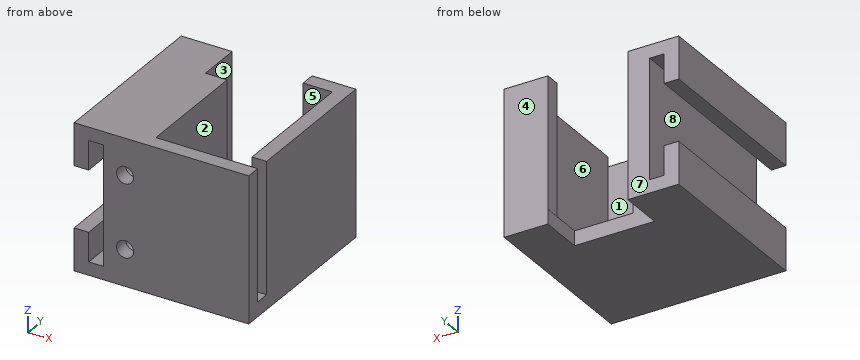
Autodesk Inventor part; units mm, degrees
ref_plane "YZ Plane" through (0, 0, 0) normal (1, 0, 0) x (0, 1, 0)
ref_plane "XZ Plane" through (0, 0, 0) normal (0, 1, 0) x (-1, 0, 0)
ref_plane "XY Plane" through (0, 0, 0) normal (0, 0, 1) x (1, 0, 0)
sketch "Sketch3" plane through (0, 0, 0) normal (0, 0, 1) x (1, 0, 0)
  line L0 (0, 0) -> (0, 60)
  line L1 (0, 60) -> (17.5, 60)
  line L2 (17.5, 60) -> (17.5, 45)
  line L3 (17.5, 45) -> (45, 45)
  line L4 (45, 45) -> (45, 60)
  line L5 (10.4377, 0) -> (0, 0)
  line L6 (45, 60) -> (60, 60)
  line L7 (60, 60) -> (60, 0)
  line L8 (60, 0) -> (0, 0)
  dimension "d7" = 60
  dimension "d8" = 17.5
  dimension "d12" = 15
  dimension "d13" = 27.5
  dimension "d14" = 15
  dimension "d15" = 60
  dimension "d16" = 60
extrude "Extrusion2" add sketch "Sketch3" along normal blind 5
sketch "Sketch4" plane through (0, 60, 0) normal (0, 1, 0) x (1, 0, 0)
  line L0 (17.5, -5) -> (0, -5)
  line L1 (0, -50) -> (17.5, -50)
  line L2 (17.5, -50) -> (17.5, -5)
  line L3 (17.5, -5) -> (0, -5)
  line L4 (0, -5) -> (0, -50)
  point P0 (0, 0)
  dimension "d20" = 45
  dimension "d21" = 17.5
extrude "Extrusion3" add sketch "Sketch4" against normal blind 60
sketch "Sketch5" plane through (45, 60, 0) normal (0, 1, 0) x (1, 0, 0)
  line L0 (15, 0) -> (15, -5)
  line L1 (-0.039, -50) -> (15, -50)
  line L2 (15, -50) -> (15, -5)
  line L3 (15, -5) -> (-0.039, -5)
  line L4 (-0.039, -5) -> (-0.039, -50)
  point P0 (-45, 0)
  dimension "d24" = 45
extrude "Extrusion4" add sketch "Sketch5" against normal blind 5
sketch "Sketch7" plane through (17.5, 45, 0) normal (0, 1, 0) x (1, 0, 0)
  line L0 (0, -5) -> (0, -50)
  line L1 (27.5, -5) -> (0, -5)
  line L2 (0, -50) -> (7.5, -50)
  line L3 (7.5, -50) -> (7.5, -5)
  line L4 (7.5, -5) -> (0, -5)
  line L5 (0, -5) -> (0, -50)
  point P0 (-17.5, 0)
  dimension "d27" = 7.5
extrude "Extrusion5" add sketch "Sketch7" against normal blind 45
sketch "Sketch8" plane through (0, 0, 5) normal (0, 0, 1) x (1, 0, 0)
  line L0 (25, 0) -> (60, 0)
  line L1 (60, 0) -> (60, 55)
  line L2 (25, 0) -> (60, 0)
  line L3 (60, 0) -> (60, 5)
  line L4 (60, 5) -> (25, 5)
  line L5 (25, 5) -> (25, 0)
  point P0 (0, 0)
  dimension "d30" = 5
extrude "Extrusion6" add sketch "Sketch8" along normal blind 45
sketch "Sketch9" plane through (0, 0, 5) normal (0, 0, 1) x (1, 0, 0)
  line L0 (60, 55) -> (45, 55)
  line L1 (60, 55) -> (55, 55)
  line L2 (55, 55) -> (55, 5)
  line L3 (55, 5) -> (60, 5)
  line L4 (60, 5) -> (60, 55)
  point P0 (0, 0)
  dimension "d33" = 50
  dimension "d34" = 5
extrude "Extrusion7" add sketch "Sketch9" along normal blind 45
sketch "Sketch10" plane through (0, 60, 0) normal (0, 1, 0) x (1, 0, 0)
  line L0 (10, -45.5) -> (5, -45.5)
  line L1 (5, -45.5) -> (5, -4.5)
  line L2 (5, -4.5) -> (10, -4.5)
  line L3 (10, -4.5) -> (10, -45.5)
  line L4 (17.5, 0) -> (17.5, -50)
  line L5 (0, 0) -> (17.5, 0)
  line L6 (0, 0) -> (0, -50)
  dimension "d45" = 5
  dimension "d46" = 41
  dimension "d47" = 7.5
  dimension "d48" = 4.5
  dimension "d49" = 5
extrude "Extrusion8" cut sketch "Sketch10" against normal blind 60
sketch "Sketch11" plane through (0, 60, 0) normal (0, 1, 0) x (1, 0, 0)
  line L0 (5, -4.5) -> (5, -45.5)
  line L1 (0, 0) -> (0, -50)
  line L2 (5, -35.5) -> (0, -35.5)
  line L3 (0, -35.5) -> (0, -14.5)
  line L4 (0, -14.5) -> (5, -14.5)
  line L5 (5, -14.5) -> (5, -35.5)
  line L6 (0, -50) -> (17.5, -50)
  dimension "d52" = 21
  dimension "d53" = 14.5
extrude "Extrusion9" cut sketch "Sketch11" against normal blind 60
sketch "Sketch12" plane through (0, 0, 0) normal (0, -1, 0) x (1, 0, 0)
  circle A0 centre (17.5, 12.5) radius 2.5
  circle A1 centre (17.5, 37.5) radius 2.5
  line L0 (10, 45.5) -> (10, 4.5)
  line L1 (0, 50) -> (60, 50)
  line L2 (60, 0) -> (0, 0)
  dimension "d56" = 5
  dimension "d57" = 5
  dimension "d58" = 7.5
  dimension "d59" = 7.5
  dimension "d60" = 12.5
  dimension "d61" = 12.5
hole "Hole1" at (17.5, 0, 12.5) at (17.5, 0, 37.5) direction (0, 1, 0) diameter 5.86 depth 5 tip angle 118
sketch "Sketch13" plane through (0, 60, 0) normal (0, 1, 0) x (1, 0, 0)
  point P0 (0, 0)
sketch "Sketch14" plane through (0, 60, 50) normal (0, 0, 1) x (1, 0, 0)
  line L0 (55, -5) -> (55, -55)
  line L1 (60, 0) -> (60, -60)
  line L2 (55, -55) -> (60, -55)
  line L3 (60, -55) -> (60, -50)
  line L4 (60, -50) -> (55, -50)
  line L5 (55, -50) -> (55, -55)
  point P0 (0, -60)
  dimension "d69" = 5
extrude "Extrusion10" cut sketch "Sketch14" against normal blind 45
sketch "Sketch15" plane through (5, 60, 35.5) normal (0, 0, -1) x (-1, 0, 0)
  point P0 (5, -60)
sketch "Sketch16" plane through (0, 60, 0) normal (0, 1, 0) x (1, 0, 0)
  point P0 (0, 0)
properties part number "Holder" material "Iron, Cast"
Design review of the part built by this model. Coordinates are the model's own, in mm. Face numbers are marked on the shaded views. A direction names the side the tool comes from. Give positions to 0.01 mm unless a question says otherwise; leave off trailing zeros. Loops run counter-clockwise (first coordinate to the right, second up) from the corner with the lowest first, then second, coordinate; pieces in that order, holes last. Notation, with made-up numbers: M 83.25,7 L 99.25,7 A13 cw 99.25,29 Z; hole C 39.25,43 d11. An arc over 180 degrees is marked long. Write item = value, one per line.
Q1. We need section C-C (y = 41). Give the boundary of the cut face in (x, z).
Output values:
outline = M 0,0 L 60,0 L 60,50 L 55,50 L 55,5 L 25,5 L 25,50 L 0,50 L 0,35.5 L 5,35.5 L 5,45.5 L 10,45.5 L 10,4.5 L 5,4.5 L 5,14.5 L 0,14.5 Z
Q2. For the marked faces 1, 2, 3, 4 and 5, list the 3-axis set-ups (+Z, -Z, +X, -X, +Y, -Y) from which the entire face can be reached by the end or side of a thin tool; tool diameter is ignored.
Output values:
face_1 = +Z, +X
face_2 = +Z, +Y
face_3 = +Z, -Z, +Y
face_4 = +Z, -Z, +X, -X, +Y
face_5 = +Z
Q3. We need section B-B (z = 24.5). Give the boundary of the cut face in (x, y).
Output values:
outline = M 10,0 L 60,0 L 60,5 L 25,5 L 25,45 L 17.5,45 L 17.5,60 L 10,60 Z; M 44.96,55 L 55,55 L 55,10 L 60,10 L 60,60 L 44.96,60 Z
Q4. We need section A-A (x = 6). Give the boundary of the cut face in (y, z).
Output values:
outline = M 0,0 L 60,0 L 60,4.5 L 0,4.5 Z; M 0,45.5 L 60,45.5 L 60,50 L 0,50 Z
Q5. Insertion check: pin 1 (12 mm diameter, centred on x = 53, y = 33.5, fed in from +Z); pin 2 (4 mm diameter, centred on y = 57.5, z = 26.5, fed in from -X); pin 3 (3.5 mm diameter, centred on x = 17.5, z = 12.5, fed in from -Y); pin 4 (2 mm diameter, centred on x = 16.5, z = 13.5, fed in from -Y). Each pin has a flat end and moves straight along its axis. Give the tip position at first contact, or say it passes through.
Output values:
pin_1 = 50
pin_2 = 10
pin_3 = 5.71
pin_4 = 5.31
Q6. To check wall thickness, follow line 1 (X direction, y = 25, z = 14); line 2 (X direction, y = 48, z = 10.5); line 3 (Z direction, x = 17.5, y = 2.3). State the ranges of each line that lie inside material, in increasing order. Write a range as [from, to].
Output values:
line_1 = [0, 5], [10, 25], [55, 60]
line_2 = [0, 5], [10, 17.5], [55, 60]
line_3 = [0, 9.57], [15.43, 34.57], [40.43, 50]
Q7. We need section D-D (x = 54). Give the boundary of the cut face in (y, z), plus the area to 3 significant figures.
Output values:
outline = M 0,0 L 60,0 L 60,50 L 55,50 L 55,5 L 5,5 L 5,50 L 0,50 Z
area = 750 mm^2
Q8. Draft analysis for pull direction Y (two halves, no side actions). For the marked faces 6, 7 and 8, state which applies: +Y half, -Y half, draft (parallel to the pull), parting line (faces both ways), or undercut.
Output values:
face_6 = undercut
face_7 = +Y half
face_8 = draft
